CAD build for the part. Positions are in the model's coordinates, mm. A direction names the side the tool comes from. Give positions to 0.01 mm unless a question says otherwise; leave off trailing zeros. Write each loop counter-clockwise with the first axis right and the second up, starting at its lowest first coordinate (ties: lowest second). Pieces come first, ordered by that corner, then holes. Notation, with made-up numbers: (70.5, 74) -> (101.5, 74) arc R35 cw to (101.5, 108) -> close; hole circle Ø5 at (84, 33.5). An arc over 180 degrees is marked (long way). Answer in a Markdown table with one row per item. Add a question column.
```python
from build123d import *

# Parameters (mm, degrees)
SKETCH2_W           = 2.54
SKETCH2_H           = 2.54
BOSS_EXTRUDE1_DEPTH = 5.08
BOSS_EXTRUDE2_DEPTH = 0.3302
LPATTERN1_COUNT     = 4
LPATTERN1_PITCH     = 2.54


with BuildPart() as part:
    # Sketch2 → Boss-Extrude1 (new, symmetric)
    with BuildSketch(Plane(origin=(0, 0, 0), x_dir=(0, 0, -1), z_dir=(1, 0, 0))):
        Rectangle(SKETCH2_W, SKETCH2_H)
    extrude(amount=BOSS_EXTRUDE1_DEPTH, both=True)

    # Sketch3 → Boss-Extrude2 (add, symmetric)
    with BuildSketch(Plane(origin=(3.81, 0, 0), x_dir=(0, 0, -1), z_dir=(1, 0, 0))):
        with BuildLine():
            Line((-0.3048, 7.112), (-0.3048, -1.778))
            ThreePointArc((-0.3048, -1.778), (-0.498226682, -2.244973318), (-0.9652, -2.4384))
            Line((-0.9652, -2.4384), (-5.103190824, -2.4384))
            Line((-5.103190824, -2.4384), (-5.103190824, -3.048))
            Line((-5.103190824, -3.048), (-0.9652, -3.048))
            ThreePointArc((-0.9652, -3.048), (-0.067174388, -2.676025612), (0.3048, -1.778))
            Line((0.3048, -1.778), (0.3048, 7.112))
            Line((0.3048, 7.112), (-0.3048, 7.112))
        make_face()
    boss_extrude2 = extrude(amount=BOSS_EXTRUDE2_DEPTH, both=True)

    # LPattern1: Boss-Extrude2 ×4
    with Locations(*[(-i * LPATTERN1_PITCH, 0, 0) for i in range(1, LPATTERN1_COUNT)]):
        add(boss_extrude2)


solid = part.part
```
Item 1: Probe L1, parallel to X at y = -2.5, z = 1.75; L2, parallel to Z at x = -3.25, y = 0.75. List the from-to ranges inside material, lowest first. Write a range as from..to.
Item 2: Drop flat-ended pins along their axis: pin 1 Ø1 at (x, y) = (-0.5, 3.5) entering from -Z; pin 2 Ø0.5 at (y, z) = (4, 0) entering from -X; pin 3 Ø0.7 at (y, z) = (4.5, 0) entering from +X; pin 4 Ø2 at (y, z) = (-0.5, 1.5) entering from +X. Give the stop position or say it passes through.
Item 3: Mould opens along X. For faces 4 (the face through (0, 0, 1.27)), 5 (the face through (5.08, 0, 0)), 6 (the face through (1.6, -2.7, 1.8)) say: released by +X, released by -X, zero draft, split by the parting line, or undercut.
Item 4: Slice it at B-B, the plane y = 3. List the corners of the cut face in (x, z), then the cut area to 3 significant figures.
Item 5: Slice it at C-C, the plane x = 3.75. List the corners of the cut face in (y, z), then the cut area to 3 significant figures.
Item 6: Slice it at A-A, the plane z = 1.5. List the corners of the cut face in (x, y), then the cut area to 3 significant figures.
Item 7: Slice it at D-D, the plane z = 0.5. List the corners of the cut face in (x, y).
Item 8: Which spindle directions (+Z, -Z, +X, -X, +Y, -Y) get a long thin tool onto all of the face, cutting with end or side? Do faces 1 (the face through (0.94, -2.7, 1.8)), 2 (the face through (-4.14, -2.7, 1.8)), 3 (the face through (4.14, -2.7, 1.8)). Say none if no direction does.
Answer key:
| question | item | result |
|---|---|---|
| 1 | L1 | x = -4.14..-3.48, -1.6..-0.94, 0.94..1.6, 3.48..4.14 |
| 1 | L2 | z = -1.27..1.27 |
| 2 | pin 1 | stops at z = -0.3 |
| 2 | pin 2 | stops at x = -4.14 |
| 2 | pin 3 | stops at x = 4.14 |
| 2 | pin 4 | stops at x = 5.08 |
| 3 | face 4 | zero draft |
| 3 | face 5 | released by +X |
| 3 | face 6 | undercut |
| 4 | outline | (-4.14, -0.3) -> (-3.48, -0.3) -> (-3.48, 0.3) -> (-4.14, 0.3) -> close; (-1.6, -0.3) -> (-0.94, -0.3) -> (-0.94, 0.3) -> (-1.6, 0.3) -> close; (0.94, -0.3) -> (1.6, -0.3) -> (1.6, 0.3) -> (0.94, 0.3) -> close; (3.48, -0.3) -> (4.14, -0.3) -> (4.14, 0.3) -> (3.48, 0.3) -> close |
| 4 | area | 1.61 mm² |
| 5 | outline | (-3.05, 0.97) arc R1.27 ccw to (-1.78, -0.3) -> (-1.27, -0.3) -> (-1.27, -1.27) -> (1.27, -1.27) -> (1.27, -0.3) -> (7.11, -0.3) -> (7.11, 0.3) -> (1.27, 0.3) -> (1.27, 1.27) -> (-1.27, 1.27) -> (-1.27, 0.3) -> (-1.78, 0.3) arc R0.66 cw to (-2.44, 0.97) -> (-2.44, 5.1) -> (-3.05, 5.1) -> close |
| 5 | area | 13.8 mm² |
| 6 | outline | (-4.14, -3.05) -> (-3.48, -3.05) -> (-3.48, -2.44) -> (-4.14, -2.44) -> close; (-1.6, -3.05) -> (-0.94, -3.05) -> (-0.94, -2.44) -> (-1.6, -2.44) -> close; (0.94, -3.05) -> (1.6, -3.05) -> (1.6, -2.44) -> (0.94, -2.44) -> close; (3.48, -3.05) -> (4.14, -3.05) -> (4.14, -2.44) -> (3.48, -2.44) -> close |
| 6 | area | 1.61 mm² |
| 7 | outline | (-5.08, -1.27) -> (5.08, -1.27) -> (5.08, 1.27) -> (-5.08, 1.27) -> close; (-4.14, -2.96) -> (-3.48, -2.96) -> (-3.48, -2.25) -> (-4.14, -2.25) -> close; (-1.6, -2.96) -> (-0.94, -2.96) -> (-0.94, -2.25) -> (-1.6, -2.25) -> close; (0.94, -2.96) -> (1.6, -2.96) -> (1.6, -2.25) -> (0.94, -2.25) -> close; (3.48, -2.96) -> (4.14, -2.96) -> (4.14, -2.25) -> (3.48, -2.25) -> close |
| 8 | face 1 | +Z, -Z, -Y |
| 8 | face 2 | +Z, -Z, -X, -Y |
| 8 | face 3 | +Z, -Z, +X, -Y |
